Geometry check sheet. Reference: the model listing, model coordinates, mm. Face numbers are marked on the shaded views. A direction names the side the tool comes from. Round coordinates to 2 decimals unless told otherwise and drop trailing zeros. Loops run counter-clockwise (first coordinate to the right, second up) from the corner with the lowest first, then second, coordinate; pieces in that order, holes last. Notation, with made-up numbers: M -38,28 L -22,28 A11 ccw -22,45 Z; hole C 31.25,62 d5. An arc over 180 degrees is marked long. Use one line per item in the form item = value. Start each with the question number.
1. Cross-section at A-A (z = 5). Record the boundary of the cut face in (x, y).
2. Draft check along X on the marked faces 5, 6 and 7. Enter one of: pulls with the +X half, pulls with the -X half, needs draft (parallel to the pull), parting line crosses it, or undercut.
3. Cross-section at B-B (y = -24.85). State how many separate pieces and enclosed holes the cut face has, then the cut area to 3 significant figures.
4. Material ranges on line 1 (Y direction, x = -10.5, z = 5); line 2 (X direction, y = -18, z = 6.75); line 3 (Y direction, x = 3.5, z = 5), recorded low to high.
5. Set-up check for the marked faces 1, 2, 3 and 4: record each of +Z, -Z, +X, -X, +Y, -Y from which the full face is reachable in a straight line by a thin tool's end or side.
6. Go/stop test with flat-tipped pins: pin 1 (1.2 mm diameter, centred on x = -9.5, z = 4.5, fed in from +Y); pin 2 (1.2 mm diameter, centred on x = -9.5, y = -21.5, fed in from +Z); pin 3 (2 mm diameter, centred on x = -9.5, z = 4.5, fed in from -Y); pin 4 (2.5 mm diameter, centred on y = -24.85, z = 5, fed in from -X). Record where each tip stops, or that it passes through.
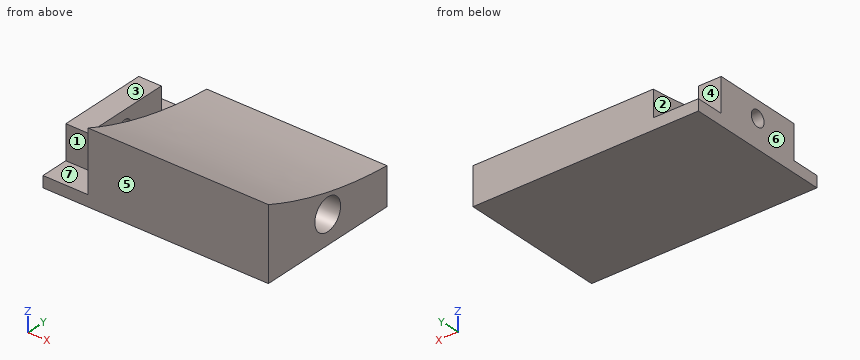
```python
from build123d import *

# Parameters (mm, degrees)
ESQUISSE1_W             = 40
ESQUISSE1_H             = 26
BOSS_EXTRU_1_DEPTH      = 2
ESQUISSE2_W             = 8
ESQUISSE2_H             = 16
BOSS_EXTRU_2_DEPTH      = 4
ESQUISSE3_R             = 1.4
ENL_V_MAT_EXTRU_1_DEPTH = 4
BOSS_EXTRU_3_DEPTH      = 32
ESQUISSE5_R             = 1.4
ENL_V_MAT_EXTRU_2_DEPTH = 41
ESQUISSE6_R             = 2.826620589
ENL_V_MAT_EXTRU_3_DEPTH = 32


with BuildPart() as part:
    # Esquisse1 → Boss.-Extru.1 (new body)
    with BuildSketch(Plane.XY):
        with Locations((8, -24.85)):
            Rectangle(ESQUISSE1_W, ESQUISSE1_H)
    extrude(amount=BOSS_EXTRU_1_DEPTH)

    # Esquisse2 → Boss.-Extru.2 (add)
    with BuildSketch(Plane.ZY.offset(12)):
        with Locations((4, -24.85)):
            Rectangle(ESQUISSE2_W, ESQUISSE2_H)
    extrude(amount=-BOSS_EXTRU_2_DEPTH)

    # Esquisse3 → Enlèv. mat.-Extru.1 (cut)
    with BuildSketch(Plane.ZY.offset(12)):
        with Locations((5, -24.85)):
            Circle(ESQUISSE3_R)
    extrude(amount=-ENL_V_MAT_EXTRU_1_DEPTH, mode=Mode.SUBTRACT)

    # Esquisse4 → Boss.-Extru.3 (add)
    with BuildSketch(Plane(origin=(28, 0, 0), x_dir=(0, 0, -1), z_dir=(1, 0, 0))):
        with BuildLine():
            Line((-6.65, -11.85), (0, -11.85))
            Line((0, -11.85), (0, -37.85))
            Line((0, -37.85), (-12.8, -37.85))
            add(Edge.make_bspline(
                [(-6.65, -11.85), (-7.550626547, -25.384236651), (-12.8, -37.85)],
                knots=[0, 0, 0, 1, 1, 1], degree=2))
        make_face()
    extrude(amount=-BOSS_EXTRU_3_DEPTH)

    # Esquisse5 → Enlèv. mat.-Extru.2 (cut)
    with BuildSketch(Plane.ZY.offset(12)):
        with Locations((5, -24.85)):
            Circle(ESQUISSE5_R)
    extrude(amount=-ENL_V_MAT_EXTRU_2_DEPTH, mode=Mode.SUBTRACT)

    # Esquisse6 → Enlèv. mat.-Extru.3 (cut)
    with BuildSketch(Plane(origin=(28, 0, 0), x_dir=(0, 0, -1), z_dir=(1, 0, 0))):
        with Locations((-5, -24.85)):
            Circle(ESQUISSE6_R)
    extrude(amount=-ENL_V_MAT_EXTRU_3_DEPTH, mode=Mode.SUBTRACT)


solid = part.part
```
Reported:
q1.outline = M -12,-32.85 L -8,-32.85 L -8,-26.25 L -12,-26.25 Z; M -12,-23.45 L -8,-23.45 L -8,-16.85 L -12,-16.85 Z; M -4,-37.85 L 28,-37.85 L 28,-27.68 L -4,-27.68 Z; M -4,-22.02 L 28,-22.02 L 28,-11.85 L -4,-11.85 Z
q2.face_5 = needs draft
q2.face_6 = pulls with the -X half
q2.face_7 = undercut
q3.separate_pieces = 3
q3.enclosed_holes = 0
q3.area = 122 mm²
q4.line_1 = -32.85 to -26.25, -23.45 to -16.85
q4.line_2 = -12 to -8, -4 to 28
q4.line_3 = -37.85 to -27.68, -22.02 to -11.85
q5.face_1 = +Z, -X, -Y
q5.face_2 = +Z, +Y, -Y
q5.face_3 = +Z, -X, +Y, -Y
q5.face_4 = +Z, -X, +Y
q6.pin_1 = -16.85
q6.pin_2 = 8
q6.pin_3 = -32.85
q6.pin_4 = through
